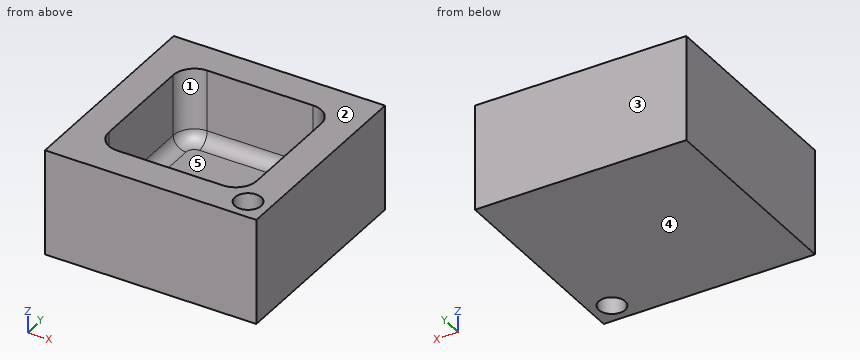
from build123d import *

# Parameters (mm, degrees)
F0_W     = 50.8
F0_H     = 25.4
F1_DEPTH = 50.8
F2_T     = -7.62
F3_R     = 5.08
F4_R     = 5.08
F5_R     = 5.08
F6_R     = 5.08
F8_D     = 6.35
F9_R     = 3.0660512242


with BuildPart() as f1:
    # F0 (on Front) → F1 (new body)
    with BuildSketch(Plane.XZ):
        with Locations((25.4, 12.7)):
            Rectangle(F0_W, F0_H)
    extrude(amount=F1_DEPTH)

    # F2
    f2_openings = [f1.faces().sort_by_distance(p)[0] for p in [
        (25.4, -25.4, 25.4),
    ]]
    offset(amount=F2_T, openings=f2_openings)

    # F3
    f3_edges = [f1.edges().sort_by_distance(p)[0] for p in [
        (7.62, -7.62, 16.51),
    ]]
    fillet(f3_edges, radius=F3_R)

    # F4
    f4_edges = [f1.edges().sort_by_distance(p)[0] for p in [
        (7.62, -43.18, 16.51),
    ]]
    fillet(f4_edges, radius=F4_R)

    # F5
    f5_edges = [f1.edges().sort_by_distance(p)[0] for p in [
        (43.18, -43.18, 16.51),
    ]]
    fillet(f5_edges, radius=F5_R)

    # F6
    f6_edges = [f1.edges().sort_by_distance(p)[0] for p in [
        (43.18, -7.62, 16.51),
    ]]
    fillet(f6_edges, radius=F6_R)

    # F8 (through all)
    with Locations(Plane.XY.offset(25.4)):
        with Locations((45.72, -45.72)):
            Hole(F8_D / 2)

    # F9
    f9_edges = [f1.edges().sort_by_distance(p)[0] for p in [
        (25.4, -7.62, 7.62),
    ]]
    fillet(f9_edges, radius=F9_R)


solid = f1.part
The listing builds one solid part. Answer for the finished solid, in the listing's coordinates (mm). Face numbers are marked on the shaded views. A direction names the side the tool comes from. Give positions to 0.01 mm unless a question says otherwise; leave off trailing zeros. Write each loop counter-clockwise with the first axis right and the second up, starting at its lowest first coordinate (ties: lowest second). Pieces come first, ordered by that corner, then holes.
1) Given P1, Ø14.5, axis at x = 20.5, y = -32, coming from the +Z side, flat-ended and moving along its own axis, determine where the tip first touches the part or whether it passes through.
2) Section D-D (x = 34.5) is taken. Write down the section's boundary in (y, z), and give its area (3 significant figures).
3) Section B-B (y = -45.72) is taken. Write down the section's boundary in (x, z) (3 decimals), and give its area (3 significant figures).
4) Section C-C (z = 16.25) is taken. Write down the section's boundary in (x, y) (3 decimals), and give its area (3 significant figures).
5) Find the intervals of material crossed by L1, parallel to Y at x = 15, z = 16; L2, parallel to Y at x = 45.5, z = 19.5; L3, parallel to X at y = -38, z = 21.5, in increasing order.
6) Section A-A (x = 45.72) is taken. Write down the section's boundary in (y, z) (3 decimals), and give its area (3 significant figures).
7) A tool of negligible diameter and unlimited length cuts with its end or side. For the marked faces 4 and 5, from which of +Z, -Z, +X, -X, +Y, -Y can it reach the whole face along a straight path? Write none if from no direction.
8) For a pull along Y with two mould halves and no side action, classify the marked faces 1, 2 and 3 as pulls with the +Y half, pulls with the -Y half, needs draft (parallel to the pull), parting line crosses it, or undercut.
Response:
1. P1: stops at z = 7.62
2. outline: (-50.8, 0) - (0, 0) - (0, 25.4) - (-7.62, 25.4) - (-7.62, 10.69) arc R3.07 cw to (-10.69, 7.62) - (-40.11, 7.62) arc R3.07 cw to (-43.18, 10.69) - (-43.18, 25.4) - (-50.8, 25.4) - close
2. area: 662 mm2
3. outline: (0, 0) - (42.545, 0) - (42.545, 25.4) - (0, 25.4) - close; (48.895, 0) - (50.8, 0) - (50.8, 25.4) - (48.895, 25.4) - close
3. area: 1,130 mm2
4. outline: (0, -50.8) - (50.8, -50.8) - (50.8, 0) - (0, 0) - close; hole (7.62, -38.1) arc R5.08 ccw to (12.7, -43.18) - (38.1, -43.18) arc R5.08 ccw to (43.18, -38.1) - (43.18, -12.7) arc R5.08 ccw to (38.1, -7.62) - (12.7, -7.62) arc R5.08 ccw to (7.62, -12.7) - close; hole circle Ø6.35 at (45.72, -45.72)
4. area: 1,310 mm2
5. L1: y = -50.8 to -43.18, -7.62 to 0
5. L2: y = -50.8 to -48.89, -42.55 to 0
5. L3: x = 0 to 7.62, 43.18 to 50.8
6. outline: (-50.8, 0) - (-48.895, 0) - (-48.895, 25.4) - (-50.8, 25.4) - close; (-42.545, 0) - (0, 0) - (0, 25.4) - (-42.545, 25.4) - close
6. area: 1,130 mm2
7. face 4: -Z, +X, -X, +Y, -Y
7. face 5: +Z
8. face 1: undercut
8. face 2: needs draft
8. face 3: pulls with the +Y half
